from build123d import *

# Parameters (mm, degrees)
BOSS_EXTRUDE1_DEPTH = 3.175


with BuildPart() as part:
    # Sketch1 → Boss-Extrude1 (new body)
    with BuildSketch(Plane(origin=(0, 0, 0), x_dir=(1, 0, 0), z_dir=(0, 1, 0))):
        Polygon((-139.430495518, 6.053301935), (-139.430495518, 2.053301935), (-134.350495518, 2.053301935), (-134.350495518, -1.121698065), (-129.270495518, -1.121698065), (-129.270495518, 2.053301935), (-124.190495518, 2.053301935), (-124.190495518, -1.121698065), (-119.110495518, -1.121698065), (-119.110495518, 2.053301935), (-114.030495518, 2.053301935), (-114.030495518, -1.121698065), (-108.950495518, -1.121698065), (-108.950495518, 2.053301935), (-103.870495518, 2.053301935), (-103.870495518, -1.121698065), (-98.790495518, -1.121698065), (-98.790495518, 2.053301935), (-93.710495518, 2.053301935), (-93.710495518, -1.121698065), (-88.630495518, -1.121698065), (-88.630495518, 2.053301935), (-83.550495518, 2.053301935), (-83.550495518, -1.121698065), (-78.470495518, -1.121698065), (-78.470495518, 2.053301935), (-73.390495518, 2.053301935), (-73.390495518, -1.121698065), (-68.310495518, -1.121698065), (-68.310495518, 2.053301935), (-63.230495518, 2.053301935), (-63.230495518, -1.121698065), (-58.150495518, -1.121698065), (-58.150495518, 2.053301935), (-53.070495518, 2.053301935), (-53.070495518, -1.121698065), (-47.990495518, -1.121698065), (-47.990495518, 2.053301935), (-42.910495518, 2.053301935), (-42.910495518, -1.121698065), (-37.830495518, -1.121698065), (-37.830495518, 2.053301935), (-32.750495518, 2.053301935), (-32.750495518, -1.121698065), (-27.670495518, -1.121698065), (-27.670495518, 2.053301935), (-22.590495518, 2.053301935), (-22.590495518, -1.121698065), (-17.510495518, -1.121698065), (-17.510495518, 2.053301935), (-12.430495518, 2.053301935), (-12.430495518, -1.121698065), (-7.350495518, -1.121698065), (-7.350495518, 2.053301935), (-2.270495518, 2.053301935), (-2.270495518, -1.121698065), (2.809504482, -1.121698065), (2.809504482, 2.053301935), (7.889504482, 2.053301935), (7.889504482, -1.121698065), (12.969504482, -1.121698065), (12.969504482, 2.053301935), (18.049504482, 2.053301935), (18.049504482, -1.121698065), (23.129504482, -1.121698065), (23.129504482, 2.053301935), (28.209504482, 2.053301935), (28.209504482, -1.121698065), (33.289504482, -1.121698065), (33.289504482, 2.053301935), (38.369504482, 2.053301935), (38.369504482, -1.121698065), (43.449504482, -1.121698065), (43.449504482, 2.053301935), (48.529504482, 2.053301935), (48.529504482, -1.121698065), (53.609504482, -1.121698065), (53.609504482, 2.053301935), (58.689504482, 2.053301935), (58.689504482, -1.121698065), (63.769504482, -1.121698065), (63.769504482, 2.053301935), (70.119504482, 2.053301935), (70.119504482, 6.053301935), (66.309504482, 6.053301935), (63.769504482, 6.053301935), (61.610504482, 11.133301935), (60.848504482, 11.133301935), (58.689504482, 6.053301935), (56.149504482, 6.053301935), (53.990504482, 11.133301935), (53.228504482, 11.133301935), (51.069504482, 6.053301935), (48.529504482, 6.053301935), (46.370504482, 11.133301935), (45.608504482, 11.133301935), (43.449504482, 6.053301935), (40.909504482, 6.053301935), (38.750504482, 11.133301935), (37.988504482, 11.133301935), (35.829504482, 6.053301935), (33.289504482, 6.053301935), (31.130504482, 11.133301935), (30.368504482, 11.133301935), (28.209504482, 6.053301935), (25.669504482, 6.053301935), (23.510504482, 11.133301935), (22.748504482, 11.133301935), (20.589504482, 6.053301935), (18.049504482, 6.053301935), (15.890504482, 11.133301935), (15.128504482, 11.133301935), (12.969504482, 6.053301935), (10.429504482, 6.053301935), (8.270504482, 11.133301935), (7.508504482, 11.133301935), (5.349504482, 6.053301935), (2.809504482, 6.053301935), (0.650504482, 11.133301935), (-0.111495518, 11.133301935), (-2.270495518, 6.053301935), (-4.810495518, 6.053301935), (-6.969495518, 11.133301935), (-7.731495518, 11.133301935), (-9.890495518, 6.053301935), (-12.430495518, 6.053301935), (-14.589495518, 11.133301935), (-15.351495518, 11.133301935), (-17.510495518, 6.053301935), (-20.050495518, 6.053301935), (-22.209495518, 11.133301935), (-22.971495518, 11.133301935), (-25.130495518, 6.053301935), (-27.670495518, 6.053301935), (-29.829495518, 11.133301935), (-30.591495518, 11.133301935), (-32.750495518, 6.053301935), (-35.290495518, 6.053301935), (-37.449495518, 11.133301935), (-38.211495518, 11.133301935), (-40.370495518, 6.053301935), (-42.910495518, 6.053301935), (-45.069495518, 11.133301935), (-45.831495518, 11.133301935), (-47.990495518, 6.053301935), (-50.530495518, 6.053301935), (-52.689495518, 11.133301935), (-53.451495518, 11.133301935), (-55.610495518, 6.053301935), (-58.150495518, 6.053301935), (-60.309495518, 11.133301935), (-61.071495518, 11.133301935), (-63.230495518, 6.053301935), (-65.770495518, 6.053301935), (-67.929495518, 11.133301935), (-68.691495518, 11.133301935), (-70.850495518, 6.053301935), (-73.390495518, 6.053301935), (-75.549495518, 11.133301935), (-76.311495518, 11.133301935), (-78.470495518, 6.053301935), (-81.010495518, 6.053301935), (-83.169495518, 11.133301935), (-83.931495518, 11.133301935), (-86.090495518, 6.053301935), (-88.630495518, 6.053301935), (-90.789495518, 11.133301935), (-91.551495518, 11.133301935), (-93.710495518, 6.053301935), (-96.250495518, 6.053301935), (-98.409495518, 11.133301935), (-99.171495518, 11.133301935), (-101.330495518, 6.053301935), (-103.870495518, 6.053301935), (-106.029495518, 11.133301935), (-106.791495518, 11.133301935), (-108.950495518, 6.053301935), (-111.490495518, 6.053301935), (-113.649495518, 11.133301935), (-114.411495518, 11.133301935), (-116.570495518, 6.053301935), (-119.110495518, 6.053301935), (-121.269495518, 11.133301935), (-122.031495518, 11.133301935), (-124.190495518, 6.053301935), (-126.730495518, 6.053301935), (-128.889495518, 11.133301935), (-129.651495518, 11.133301935), (-131.810495518, 6.053301935), (-134.350495518, 6.053301935), (-136.509495518, 11.133301935), (-137.271495518, 11.133301935), align=None)
    extrude(amount=BOSS_EXTRUDE1_DEPTH)


solid = part.part
The model under review builds one solid part; all positions refer to its coordinate system, in mm. A direction names the side the tool comes from. Coordinates: 2 decimals unless noted, no trailing zeros. Answer as a JSON object with one key per item and string values. Group by question number.
1. To check wall thickness, follow probe 1 along Z at (x, y) = (-81, 2.65); probe 2 along Z at (x, y) = (-118, 1). State the ranges of each line that lie inside material, in increasing order.
2. Clearance check with flat-ended pins moving along their axes: pin 1 Ø1 at (y, z) = (1, -1) entering from +X; pin 2 Ø1.3 at (x, y) = (-10.5, 2.5) entering from -Z; pin 3 Ø1 at (y, z) = (2, -1) entering from -X. State where each tip first meets the part, or that it passes through.
3. Mouldability with a two-part tool opening along X and no side actions: class faces 1 (the face through (-98.79, 2, 0)), 2 (the face through (63.77, 2, 0)), 3 (the face through (61, 2, 1.122)) as pulls with the +X half, pulls with the -X half, needs draft (parallel to the pull), parting line crosses it, or undercut.
4. Machinability: for faces 4 (the face through (-59, 0, -5)), 5 (the face through (29.304, 1.565, -8.629)), 6 (the face through (-25, 2, -2.053)), which of the approach directions +Z, -Z, +X, -X, +Y, -Y give a long, thin tool a straight path to every point of the face, cutting with its end or side? Answer none if there is none.
Findings:
{
 "1": {"probe 1": "-6.05 to 1.12", "probe 2": "-6.05 to -2.05"},
 "2": {"pin 1": "x = 63.77", "pin 2": "z = -6.15", "pin 3": "x = -134.35"},
 "3": {"face 1": "undercut", "face 2": "pulls with the +X half", "face 3": "needs draft"},
 "4": {"face 4": "+Z, -Z, +X, -X, -Y", "face 5": "-Z, +Y, -Y", "face 6": "+Z, +Y, -Y"}
}
